```python
from build123d import *

# Parameters (mm, degrees)
F0_W     = 260.35
F0_H     = 19.05
F1_DEPTH = 152.4
F2_W     = 12.7
F2_H     = 114.3
F3_DEPTH = 12.7
F4_R     = 6.34999
F5_W     = 12.7
F5_H     = 114.3
F6_DEPTH = 12.7
F7_R     = 6.34999


# Not quite as in the source:
# - a fillet or chamfer is up to 0.001 mm smaller than in the source, because OpenCascade refuses the exact size


with BuildPart() as f1:
    # F0 (on Top) → F1 (new body)
    with BuildSketch(Plane.XY):
        Rectangle(F0_W, F0_H)
    extrude(amount=-F1_DEPTH)

    # F2 (on face) → F3 (join)
    with BuildSketch(Plane(origin=(-130.175, 0, 0), x_dir=(0, -1, 0), z_dir=(-1, 0, 0))):
        with Locations((0, -76.2)):
            Rectangle(F2_W, F2_H)
    extrude(amount=F3_DEPTH)

    # F4 (radius 6.35 in the source; OpenCascade refuses exactly that, so slightly less here)
    f4_edges = [f1.edges().sort_by_distance(p)[0] for p in [
        (-136.525, 6.35, -19.05),
        (-136.525, -6.35, -19.05),
        (-136.525, -6.35, -133.35),
        (-136.525, 6.35, -133.35),
    ]]
    fillet(f4_edges, radius=F4_R)

    # F5 (on face) → F6 (join)
    with BuildSketch(Plane.YZ.offset(130.175)):
        with Locations((0, -76.2)):
            Rectangle(F5_W, F5_H)
    extrude(amount=F6_DEPTH)

    # F7 (radius 6.35 in the source; OpenCascade refuses exactly that, so slightly less here)
    f7_edges = [f1.edges().sort_by_distance(p)[0] for p in [
        (136.525, -6.35, -19.05),
        (136.525, 6.35, -19.05),
        (136.525, 6.35, -133.35),
        (136.525, -6.35, -133.35),
    ]]
    fillet(f7_edges, radius=F7_R)


solid = f1.part
```
CAD build for the part. Positions are in the model's coordinates, mm. A direction names the side the tool comes from. Coordinates: 2 decimals unless noted, no trailing zeros. Order: outer loops, then holes, each group sorted by start corner. A loop starts at its lowest first (then second) coordinate and runs counter-clockwise, first axis right, second up. Notation, with made-up numbers: (45, 45) - (93, 45) arc R19 ccw to (93, 57) - close; hole circle Ø5 at (23.5, 73.25). An arc over 180 degrees is marked (long way). Answer in a Markdown table with one row per item.
1. 3-axis set-ups, long thin cutter, end or side, ignore diameter. For faces 1 (the face through (-136.61, 4.54, -20.96)), 2 (the face through (-136, 6.35, -77)), 3 (the face through (136.61, 4.54, -20.96)): which of +Z, -Z, +X, -X, +Y, -Y reach the whole face in a straight line?
Answer:
| item | result |
|---|---|
| face 1 | +Z, -X, +Y |
| face 2 | +Z, -Z, -X, +Y |
| face 3 | +Z, +X, +Y |
2. Flat gauge pins, fed straight in: P1, Ø10, axis at x = -135.5, z = -68.5, coming from the +Y side; P2, Ø10, axis at x = -136, z = -66, coming from the -Y side. Where does each tip first touch, or does it go through?
Answer:
| item | result |
|---|---|
| P1 | y = 6.35 |
| P2 | y = -6.35 |
3. Slice it at B-B, the plane z = -121. List the corners of the cut face in (x, y) (3 decimals), then the cut area to 3 significant figures.
Answer:
| item | result |
|---|---|
| outline | (-142.875, -6.35) - (-130.175, -6.35) - (-130.175, -9.525) - (130.175, -9.525) - (130.175, -6.35) - (142.875, -6.35) - (142.875, 6.35) - (130.175, 6.35) - (130.175, 9.525) - (-130.175, 9.525) - (-130.175, 6.35) - (-142.875, 6.35) - close |
| area | 5,280 mm² |
4. Slice it at A-A, the plane y = -3. List the corners of the cut face in (x, z) (3 decimals).
Answer:
| item | result |
|---|---|
| outline | (-142.875, -132.597) - (-130.175, -132.597) - (-130.175, -152.4) - (130.175, -152.4) - (130.175, -132.597) - (142.875, -132.597) - (142.875, -19.803) - (130.175, -19.803) - (130.175, 0) - (-130.175, 0) - (-130.175, -19.803) - (-142.875, -19.803) - close |
5. Drill centre line: L1, parallel to X at y = -2.5, z = -136.5 (3 decimals). Where is it in solid material? Low to high. Write a range as from..to.
Answer:
| item | result |
|---|---|
| L1 | -130.175..130.175 |
